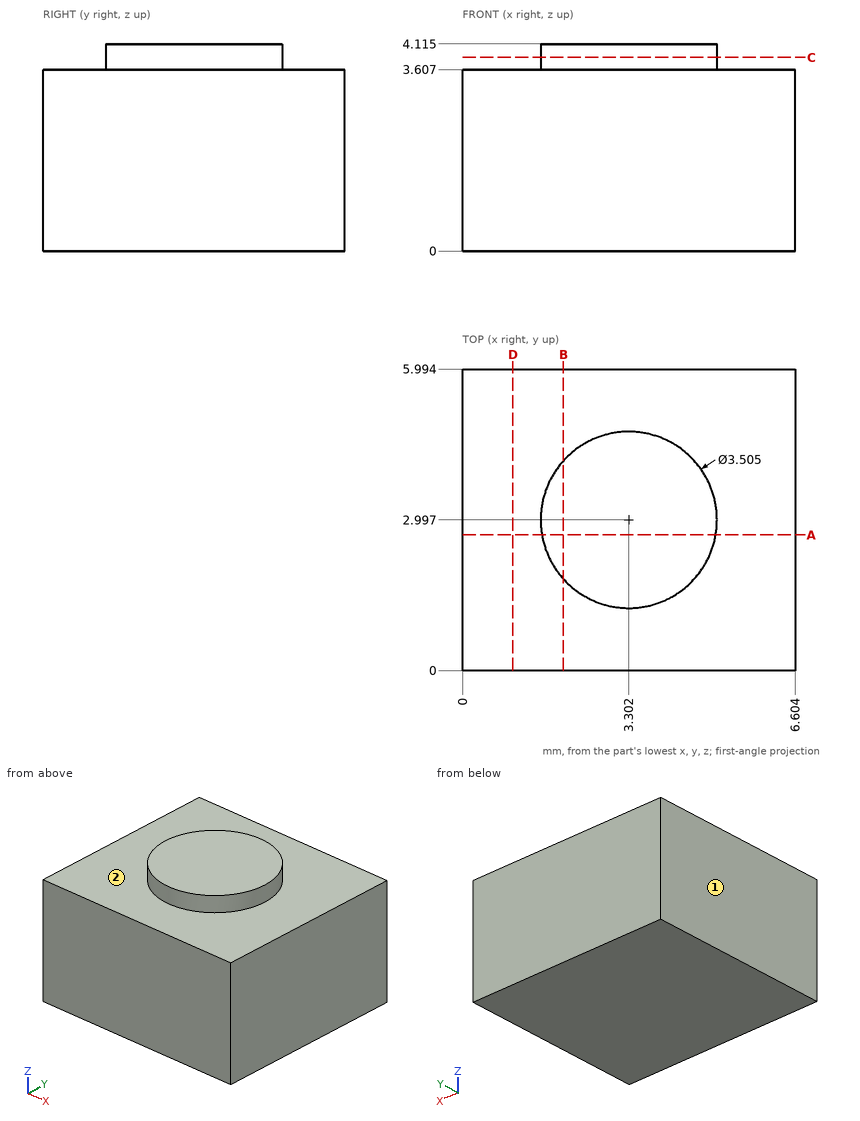
Verification items for this drawing (mm, ordinates from the low corner). A direction names the side the tool comes from. Coordinates: 2 decimals unless noted, no trailing zeros. Order: outer loops, then holes, each group sorted by start corner. A loop starts at its lowest first (then second) coordinate and runs counter-clockwise, first axis right, second up. Notation, with made-up numbers: (-36, 53.5) -> (-6, 53.5) arc R11 cw to (-6, 62.5) -> close; hole circle Ø3 at (84, 30). An arc over 180 degrees is marked (long way). Answer as CSV lines item,"result". Start each with the question number.
1) Cross-section at B-B, the plane x = 2. Record the boundary of the cut face in (y, z) (1 decimal).
2) Gauge pin test, flat end, axial feed: pin 1 Ø1 at (x, y) = (5.5, 4) entering from +Z. Record the tip position at first contact, or that the pin passes through.
3) Cross-section at C-C, the plane z = 3.85. Record the boundary of the cut face in (x, y) (1 decimal).
4) Set-up check for the marked faces 1 and 2: record each of +Z, -Z, +X, -X, +Y, -Y from which the full face is reachable in a straight line by a thin tool's end or side.
5) Cross-section at D-D, the plane x = 1. Record the boundary of the cut face in (y, z) (1 decimal), then the cut area to 3 significant figures.
6) Cross-section at A-A, the plane y = 2.7. Record the boundary of the cut face in (x, z) (1 decimal).
7) Material ranges on L1, parallel to Z at x = 4, y = 4.7, recorded low to high. Write a range as [from, to].
Conclusion:
1,outline,"(0, 0) -> (6, 0) -> (6, 3.6) -> (4.2, 3.6) -> (4.2, 4.1) -> (1.8, 4.1) -> (1.8, 3.6) -> (0, 3.6) -> close"
2,pin 1,"stops at z = 3.61"
3,outline,"circle Ø3.5 at (3.3, 3)"
4,face 1,"+Z, -Z, -X, +Y, -Y"
4,face 2,"+Z"
5,outline,"(0, 0) -> (6, 0) -> (6, 3.6) -> (0, 3.6) -> close"
5,area,"21.6 mm²"
6,outline,"(0, 0) -> (6.6, 0) -> (6.6, 3.6) -> (5, 3.6) -> (5, 4.1) -> (1.6, 4.1) -> (1.6, 3.6) -> (0, 3.6) -> close"
7,L1,"z = [0, 3.61]"
